```python
from build123d import *

# Parameters (mm, degrees)
F1_DEPTH = 248.031
F3_D     = 3.6


with BuildPart() as f1:
    # F0 (on Right) → F1 (new body)
    with BuildSketch(Plane.YZ):
        Polygon((0, 76.8765774002), (0, 0), (183.261, 0), (183.261, 38.1), (119.5924225998, 91.694), (14.8174225998, 91.694), align=None)
    extrude(amount=F1_DEPTH)

    # F3 (through all)
    with Locations(Plane.YZ.offset(248.031)):
        with Locations((21.59, 84.455), (6.985, 70.485), (6.985, 31.75), (175.895, 31.75), (114.554, 84.455)):
            Hole(F3_D / 2)


solid = f1.part
```
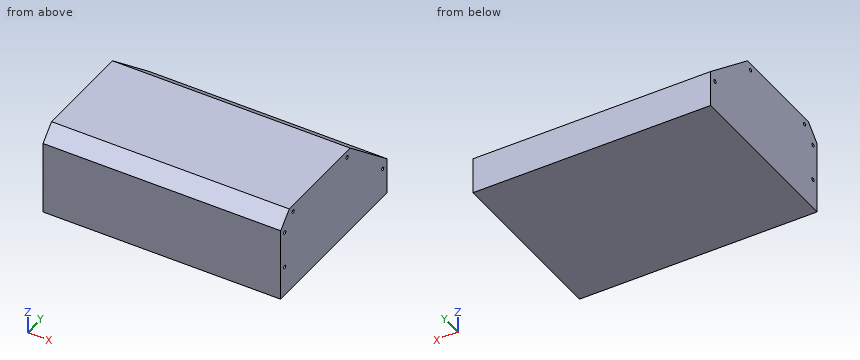
The listing builds one solid part. Answer for the finished solid, in the listing's coordinates (mm). Give positions to 0.01 mm unless a question says otherwise; leave off trailing zeros. Order: outer loops, then holes, each group sorted by start corner. A loop starts at its lowest first (then second) coordinate and runs counter-clockwise, first axis right, second up.
Item 1: The part is cut by section C-C, the plane z = 64.5. Give the vertices of the cut face in (x, y), and give its area (3 significant figures).
From the geometry:
outline: (0, 0) - (248.03, 0) - (248.03, 151.9) - (0, 151.9) - close
area: 37,700 mm2
Item 2: Find the intervals of material crossed by probe 1 along Y at (x, z) = (100, 31); probe 2 along Y at (x, z) = (124, 48); probe 3 along Y at (x, z) = (90, 63), in increasing order.
From the geometry:
probe 1: y = 0 to 5.35, 8.62 to 174.26, 177.53 to 183.26
probe 2: y = 0 to 171.5
probe 3: y = 0 to 153.68
Item 3: Given pin 1 Ø1.5 at (x, z) = (58, 52) entering from +Y, flat-ended and moving along its own axis, determine where the tip first touches the part or whether it passes through.
From the geometry:
pin 1: stops at y = 167.64
Item 4: The part is cut by section B-B, the plane z = 48. Give the vertices of the cut face in (x, y), and give its area (3 significant figures).
From the geometry:
outline: (0, 0) - (248.03, 0) - (248.03, 171.5) - (0, 171.5) - close
area: 42,500 mm2
Item 5: The part is cut by section A-A, the plane x = 82. Give the vertices of the cut face in (y, z) (3 decimals), and give its area (3 significant figures).
From the geometry:
outline: (0, 0) - (183.261, 0) - (183.261, 38.1) - (119.592, 91.694) - (14.817, 91.694) - (0, 76.877) - close; hole circle Ø3.6 at (6.985, 31.75); hole circle Ø3.6 at (6.985, 70.485); hole circle Ø3.6 at (21.59, 84.455); hole circle Ø3.6 at (114.554, 84.455); hole circle Ø3.6 at (175.895, 31.75)
area: 14,900 mm2
